from build123d import *

# Parameters (mm, degrees)
F1_DEPTH  = 102
F2_R      = 50.99999
F3_R      = 27
F3_R_2    = 18.5
F4_DEPTH  = 30
F8_DEPTH  = 10
F5_R      = 10
F9_DEPTH  = 30
F10_R     = 18.5
F11_DEPTH = 30
F12_R     = 20
F13_R     = 20


# Not quite as in the source:
# - a fillet or chamfer is up to 0.001 mm smaller than in the source, because OpenCascade refuses the exact size


with BuildPart() as f1:
    # F0 (on Top) → F1 (new body)
    with BuildSketch(Plane.XY):
        Polygon((-3.5224159509, -94.9145984159), (-111.5168624514, 92.1372698583), (-134.0335229498, 79.1372698583), (-18.5335229498, -120.9145984159), (105.4775840491, -120.9145984159), (105.4775840491, -94.9145984159), align=None)
    extrude(amount=F1_DEPTH)

    # F2 (radius 51 in the source; OpenCascade refuses exactly that, so slightly less here)
    f2_edges = [f1.edges().sort_by_distance(p)[0] for p in [
        (-122.775193, 85.63727, 102),
        (-122.775193, 85.63727, 0),
    ]]
    fillet(f2_edges, radius=F2_R)

    # F3 (on face) → F4 (join)
    with BuildSketch(Plane(origin=(-43.7410386722, -25.253900452, 0), x_dir=(-0.5, 0.8660254038, 0), z_dir=(0.8660254038, 0.5, 0))):
        with Locations((84.5516475584, 51)):
            Circle(F3_R)
        with Locations((84.5516475584, 51)):
            Circle(F3_R_2, mode=Mode.SUBTRACT)
    extrude(amount=F4_DEPTH)

    # F7 (on offset) → F8 (join, symmetric)
    with BuildSketch(Plane.XY.offset(51)):
        Polygon((-3.5224159509, -94.9145984159), (105.4775840491, -94.9145984159), (-44.2564783831, -30.7528017003), align=None)
    extrude(amount=F8_DEPTH, both=True)

    # F5 (on face) → F9 (cut)
    with BuildSketch(Plane(origin=(0, -94.9145984159, 0), x_dir=(-1, 0, 0), z_dir=(0, 1, 0))):
        with Locations((-85.4775840491, 82)):
            Circle(F5_R)
        with Locations((-85.4775840491, 20)):
            Circle(F5_R)
        with Locations((-16.4775840491, 82)):
            Circle(F5_R)
        with Locations((-16.4775840491, 20)):
            Circle(F5_R)
    extrude(amount=-F9_DEPTH, mode=Mode.SUBTRACT)

    # F10 (on face) → F11 (cut)
    with BuildSketch(Plane(origin=(-43.7410386722, -25.253900452, 0), x_dir=(-0.5, 0.8660254038, 0), z_dir=(0.8660254038, 0.5, 0))):
        with Locations((84.5516475584, 51)):
            Circle(F10_R)
    extrude(amount=-F11_DEPTH, mode=Mode.SUBTRACT)

    # F12
    f12_edges = [f1.edges().sort_by_distance(p)[0] for p in [
        (105.477584, -107.914598, 102),
    ]]
    fillet(f12_edges, radius=F12_R)

    # F13
    f13_edges = [f1.edges().sort_by_distance(p)[0] for p in [
        (105.477584, -107.914598, 0),
    ]]
    fillet(f13_edges, radius=F13_R)


solid = f1.part
Input: part model. Units: mm. Frame: model coordinates. A direction names the side the tool comes from. Coordinates: 2 decimals unless noted, no trailing zeros. Order: outer loops, then holes, each group sorted by start corner. A loop starts at its lowest first (then second) coordinate and runs counter-clockwise, first axis right, second up. Notation, with made-up numbers: M -10.75,-39.75 L 17.25,-39.75 A20 cw 17.25,-3.75 Z; hole C -20.5,2 d8. An arc over 180 degrees is marked long. Write item = value, one per line. Start each with the question number.
(1) Section B-B on y = -45.5. Output: boundary loops of the cut face in (x, z), and give its area (3 significant figures).
(2) Section A-A on z = 66.5. Output: boundary loops of the cut face in (x, y).
(3) Reachability of faces 1 (the flat face through (22, -75, 41)), 2 (the flat face through (22, -75, 61)), 3 (the flat face through (-56.85, 57.45, 33.38)) from +Z, -Z, +X, -X, +Y, -Y: full face, straight path, thin tool, end or side. Return the list, or none.
(4) Section C-C on x = 63.5. Output: boundary loops of the cut face in (y, z).
(5) Pull-direction query (X, two-part tool) for faces 4 (the flat face through (-77.09, -19.49, 50.29)), 5 (the cylindrical face through (86.779, -107.733, 91.915)), 6 (the cylindrical face through (80.1, -107.73, 28.43)), 7 (the flat face through (52, -94.915, 20)); classes: released by +X, released by -X, zero draft, split by the parting line, or undercut.
(6) Section D-D on z = 95. Output: boundary loops of the cut face in (x, y), and give its area (3 significant figures).
(7) First-contact query: P1, Ø12.5, axis at x = 50.5, z = 90.5, coming from the +Y side; P2, Ø18.5, axis at x = 63.5, y = -70, coming from the +Z side; P3, Ø6, axis at y = -3, z = 47.5, coming from the +X side; P4, Ø12, axis at x = 16.48, z = 82, coming from the +Y side. Flat tips, straight axial feed; report the tip coordinate or a pass-through.
(8) Line query: line 1 along Y through (x, z) = (66, 95); line 2 along Z through (x, y) = (-56.5, 53); line 3 along Y through (x, z) = (-90.5, 40) (3 decimals). Output: solid intervals per line, ascending. Write a range as [from, to].
Result set:
q1.outline = M -62.07,0 L -32.05,0 L -32.05,41 L -9.84,41 L -9.84,61 L -32.05,61 L -32.05,102 L -62.07,102 Z
q1.area = 3,510 mm²
q2.outline = M -132.83,77.05 L -113.58,43.72 L -65.09,71.72 L -71.09,82.12 L -97.07,67.12 L -110.31,90.05 Z; M -103.48,26.22 L -18.53,-120.91 L 105.48,-120.91 L 105.48,-94.91 L -3.52,-94.91 L -74.96,28.82 L -48.98,43.82 L -54.99,54.22 Z
q3.face_1 = -Z, +X, +Y
q3.face_2 = +Z, +X, +Y
q3.face_3 = +Z, -Z, +X, +Y
q4.outline = M -120.91,0 L -94.91,0 L -94.91,41 L -76.93,41 L -76.93,61 L -94.91,61 L -94.91,102 L -120.91,102 Z
q5.face_4 = released by -X
q5.face_5 = undercut
q5.face_6 = undercut
q5.face_7 = zero draft
q6.outline = M -121.43,57.3 L -18.53,-120.91 L 100.68,-120.91 L 100.68,-94.91 L -3.52,-94.91 L -98.91,70.3 Z
q6.area = 8,060 mm²
q7.P1 = -94.91
q7.P2 = 61
q7.P3 = -54.86
q7.P4 = through
q8.line_1 = [-120.91, -94.91]
q8.line_2 = [26.08, 35.7], [66.3, 75.92]
q8.line_3 = [3.735, 28.206], [62.557, 73.854]
